```python
from build123d import *

# Parameters (mm, degrees)
SKETCH1_W           = 37
SKETCH1_H           = 11.7
BOSS_EXTRUDE1_DEPTH = 69
CUT_EXTRUDE1_DEPTH  = 67
SKETCH3_W           = 20
SKETCH3_H           = 5.9
CUT_EXTRUDE2_DEPTH  = 67
BOSS_EXTRUDE2_START = -34
SKETCH4_R           = 1.9
BOSS_EXTRUDE2_DEPTH = 3
FILLET1_R           = 2
SKETCH5_W           = 3.5
SKETCH5_H           = 9
CUT_EXTRUDE3_DEPTH  = 40
BOSS_EXTRUDE3_START = 0.5
BOSS_EXTRUDE3_DEPTH = 2.5


with BuildPart() as part:
    # Sketch1 → Boss-Extrude1 (new body)
    with BuildSketch(Plane(origin=(0, 0, 0), x_dir=(1, 0, 0), z_dir=(0, 1, 0))):
        with Locations((18.5, 5.85)):
            Rectangle(SKETCH1_W, SKETCH1_H)
    extrude(amount=BOSS_EXTRUDE1_DEPTH)

    # Sketch2 → Cut-Extrude1 (cut)
    with BuildSketch(Plane(origin=(0, 69, 0), x_dir=(1, 0, 0), z_dir=(0, 1, 0))):
        Polygon((3, 0), (3, 2), (2, 2), (2, 3.8), (3, 3.8), (3, 9.7), (34, 9.7), (34, 3.8), (35, 3.8), (35, 2), (34, 2), (34, 0), align=None)
    extrude(amount=-CUT_EXTRUDE1_DEPTH, mode=Mode.SUBTRACT)

    # Sketch3 → Cut-Extrude2 (cut)
    with BuildSketch(Plane(origin=(0, 2, 0), x_dir=(1, 0, 0), z_dir=(0, 1, 0))):
        with Locations((19.275, 6.75)):
            Rectangle(SKETCH3_W, SKETCH3_H)
    extrude(amount=-CUT_EXTRUDE2_DEPTH, mode=Mode.SUBTRACT)

    # Sketch4 → Boss-Extrude2 (add)
    # profile 1 of 2: a face of its own
    with BuildSketch(Plane(origin=(37, 0, 0), x_dir=(0, 0, -1), z_dir=(1, 0, 0)).offset(BOSS_EXTRUDE2_START)):
        with BuildLine():
            Line((11.7, 63.35), (19.7, 63.35))
            ThreePointArc((19.7, 63.35), (23.6, 59.45), (19.7, 55.55))
            Line((19.7, 55.55), (11.7, 55.55))
            Line((11.7, 55.55), (11.7, 63.35))
        make_face()
        with Locations((19.7, 59.45)):
            Circle(SKETCH4_R, mode=Mode.SUBTRACT)
    # profile 2 of 2: a face of its own
    with BuildSketch(Plane(origin=(37, 0, 0), x_dir=(0, 0, -1), z_dir=(1, 0, 0)).offset(BOSS_EXTRUDE2_START)):
        with BuildLine():
            Line((11.7, 27.35), (19.7, 27.35))
            ThreePointArc((19.7, 27.35), (23.6, 23.45), (19.7, 19.55))
            Line((19.7, 19.55), (11.7, 19.55))
            Line((11.7, 19.55), (11.7, 27.35))
        make_face()
        with Locations((19.7, 23.45)):
            Circle(SKETCH4_R, mode=Mode.SUBTRACT)
    extrude(amount=-BOSS_EXTRUDE2_DEPTH)

    # Fillet1
    fillet1_edges = [part.edges().sort_by_distance(p)[0] for p in [
        (1.5, 55.55, -11.7),
        (1.5, 63.35, -11.7),
        (3, 59.45, -11.7),
        (1.5, 19.55, -11.7),
        (1.5, 27.35, -11.7),
        (3, 23.45, -11.7),
    ]]
    fillet(fillet1_edges, radius=FILLET1_R)

    # Sketch5 → Cut-Extrude3 (cut)
    with BuildSketch(Plane(origin=(37, 0, 0), x_dir=(0, 0, -1), z_dir=(1, 0, 0))):
        with Locations((3.25, 6.5)):
            Rectangle(SKETCH5_W, SKETCH5_H)
    extrude(amount=-CUT_EXTRUDE3_DEPTH, mode=Mode.SUBTRACT)

    # Sketch6 → Boss-Extrude3 (add)
    with BuildSketch(Plane.XY.offset(-5).offset(BOSS_EXTRUDE3_START)):
        with BuildLine():
            Line((37, 2), (37, 9.5))
            Line((37, 9.5), (35.75, 9.5))
            ThreePointArc((35.75, 9.5), (34.689339828, 9.060660172), (34.25, 8))
            Line((34.25, 8), (34.25, 7.5))
            ThreePointArc((34.25, 7.5), (34.542893219, 6.792893219), (35.25, 6.5))
            Line((35.25, 6.5), (35.25, 2))
            Line((35.25, 2), (37, 2))
        make_face()
    boss_extrude3 = extrude(amount=BOSS_EXTRUDE3_DEPTH)

    # Mirror1: Boss-Extrude3 across plane
    add(boss_extrude3.mirror(Plane(origin=(18.5, 0, 0), x_dir=(0, 0, 1), z_dir=(1, 0, 0))))


solid = part.part
```
CAD build for the part. Positions are in the model's coordinates, mm. A direction names the side the tool comes from. Give positions to 0.01 mm unless a question says otherwise; leave off trailing zeros. Loops run counter-clockwise (first coordinate to the right, second up) from the corner with the lowest first, then second, coordinate; pieces in that order, holes last. Notation, with made-up numbers: (-8.5, 18.5) -> (6.5, 18.5) arc R28 ccw to (6.5, 44.5) -> close; hole circle Ø3 at (9, 68.25). An arc over 180 degrees is marked (long way). Use a Markdown table: item, result.
1. Slice it at B-B (y = 5). List the corners of the cut face in (x, z).
Check result:
| item | result |
|---|---|
| outline | (0, -11.7) -> (37, -11.7) -> (37, -5) -> (34, -5) -> (34, -9.7) -> (3, -9.7) -> (3, -5) -> (0, -5) -> close; (0, -4.5) -> (1.75, -4.5) -> (1.75, -2) -> (0, -2) -> close; (0, -1.5) -> (3, -1.5) -> (3, 0) -> (0, 0) -> close; (34, -1.5) -> (37, -1.5) -> (37, 0) -> (34, 0) -> close; (35.25, -4.5) -> (37, -4.5) -> (37, -2) -> (35.25, -2) -> close |
2. Slice it at A-A (z = -3). List the corners of the cut face in (x, y), plus the area to 3 significant figures.
Check result:
| item | result |
|---|---|
| outline | (0, 0) -> (37, 0) -> (37, 9.5) -> (35.75, 9.5) arc R1.5 ccw to (34.25, 8) -> (34.25, 7.5) arc R1 ccw to (35.25, 6.5) -> (35.25, 2) -> (1.75, 2) -> (1.75, 6.5) arc R1 ccw to (2.75, 7.5) -> (2.75, 8) arc R1.5 ccw to (1.25, 9.5) -> (0, 9.5) -> close; (0, 11) -> (2, 11) -> (2, 69) -> (0, 69) -> close; (35, 11) -> (37, 11) -> (37, 69) -> (35, 69) -> close |
| area | 337 mm^2 |
3. Slice it at C-C (x = 17). List the corners of the cut face in (y, z), plus the area to 3 significant figures.
Check result:
| item | result |
|---|---|
| outline | (0, -11.7) -> (69, -11.7) -> (69, -9.7) -> (0, -9.7) -> close; (0, -3.8) -> (2, -3.8) -> (2, 0) -> (0, 0) -> close |
| area | 146 mm^2 |
4. Flat gauge pins, fed straight in: pin 1 (3 mm diameter, centred on x = 1, y = 4, fed in from -Z); pin 2 (9.5 mm diameter, centred on x = 22.5, y = 26.5, fed in from +Z); pin 3 (2.5 mm diameter, centred on x = 1, z = -15.5, fed in from +Y). Where does each tip first touch, or does it go through?
Check result:
| item | result |
|---|---|
| pin 1 | stops at z = -11.7 |
| pin 2 | stops at z = -9.7 |
| pin 3 | stops at y = 63.35 |
5. Mould opens along Y. For faces 1 (the flat face through (36, 6, -5)), 2 (the flat face through (2, 40, -3)), 3 (the flat face through (18, 0, -3)) say: pulls with the +Y half, pulls with the -Y half, needs draft (parallel to the pull), parting line crosses it, or undercut.
Check result:
| item | result |
|---|---|
| face 1 | undercut |
| face 2 | needs draft |
| face 3 | pulls with the -Y half |
6. Which spindle directions (+Z, -Z, +X, -X, +Y, -Y) get a long thin tool onto all of the face, cutting with end or side? Do faces 4 (the flat face through (3, 23.5, -17.6)), 5 (the flat face through (34, 36, -1)), 6 (the flat face through (1, 6, -2)). Say none if no direction does.
Check result:
| item | result |
|---|---|
| face 4 | -Z, +X, +Y, -Y |
| face 5 | +Z, +Y |
| face 6 | +X, -X |
7. Wall check: L1, parallel to Y at x = 1.75, z = -19.7; L2, parallel to X at y = 55.5, z = -6.25; L3, parallel to X at y = 27.5, z = -3.75. Give the ranges that are in metal, low to high. Write a range as [from, to].
Check result:
| item | result |
|---|---|
| L1 | y = [19.55, 21.55], [25.35, 27.35], [55.55, 57.55], [61.35, 63.35] |
| L2 | x = [0, 3], [34, 37] |
| L3 | x = [0, 2], [35, 37] |
8. Slice it at D-D (z = -14.5). List the corners of the cut face in (x, y), plus the area to 3 significant figures.
Check result:
| item | result |
|---|---|
| outline | (0, 19.55) -> (3, 19.55) -> (3, 27.35) -> (0, 27.35) -> close; (0, 55.55) -> (3, 55.55) -> (3, 63.35) -> (0, 63.35) -> close |
| area | 46.8 mm^2 |
